Design review of the part built by this model. Coordinates are the model's own, in mm. A direction names the side the tool comes from. Coordinates: 2 decimals unless noted, no trailing zeros. Order: outer loops, then holes, each group sorted by start corner. A loop starts at its lowest first (then second) coordinate and runs counter-clockwise, first axis right, second up. Notation, with made-up numbers: (-33, 51) -> (5, 51) arc R23 ccw to (5, 69) -> close; hole circle Ø10 at (7.25, 44). An arc over 180 degrees is marked (long way). Write item = value, one per line.
Autodesk Inventor part; units mm, degrees
ref_plane "Work Plane1" through (0, 0, 48) normal (0, 0, 1) x (1, 0, 0)
ref_plane "YZ Plane" through (0, 0, 0) normal (1, 0, 0) x (0, 1, 0)
ref_plane "XZ Plane" through (0, 0, 0) normal (0, 1, 0) x (-1, 0, 0)
sketch "Sketch1" plane through (0, 0, 0) normal (0, 0, 1) x (1, 0, 0)
  line L0 (-19.05, 19.05) -> (19.05, 19.05)
  line L1 (19.05, 19.05) -> (19.05, -19.05)
  line L2 (19.05, -19.05) -> (-19.05, -19.05)
  line L3 (-19.05, -19.05) -> (-19.05, 19.05)
  point P0 (0, 0)
  point P1 (-19.05, 0)
  point P2 (0, 19.05)
  dimension "d0" = 38.1
extrude "Extrusion1" add sketch "Sketch1" along normal blind 56
sketch "Sketch2" plane through (-19.05, 19.05, 0) normal (0, 1, 0) x (1, 0, 0)
  circle A0 centre (19.05, -28) radius 12.7
  line L0 (0, 0) -> (38.1, 0)
  line L1 (0, -56) -> (38.1, -56)
  line L2 (17.05, 0) -> (21.05, 0)
  line L3 (21.05, 0) -> (21.05, -28)
  line L4 (21.05, -28) -> (17.05, -28)
  line L5 (17.05, -28) -> (17.05, 0)
  point P0 (19.05, 0)
  dimension "d3" = 28
  dimension "d4" = 25.4
  dimension "d5" = 4
extrude "Extrusion2" cut sketch "Sketch2" against normal through all
ref_plane "Work Plane1" through (0, 0, 48) normal (0, 0, 1) x (1, 0, 0)
sketch "Sketch3" plane through (0, 0, 48) normal (0, 0, 1) x (1, 0, 0)
  point P0 (0, 0)
hole "Hole1" at (0, 0, 48) direction (0, 0, 1) diameter 9 end through all
sketch "Sketch4" plane through (0, 0, 0) normal (0, 0, -1) x (-1, 0, 0)
  circle A0 centre (0, 0) radius 8
  dimension "d16" = 16
extrude "Extrusion3" cut sketch "Sketch4" against normal up to surface (48 mm away)
sketch "Sketch5" plane through (-19.05, -19.05, 0) normal (-1, 0, 0) x (0, 0, 1)
  line L0 (0, 0) -> (0, 38.1)
  circle A0 centre (5.7121, 19.05) radius 3.8228
  line L1 (4.9053, 27.6435) -> (6.5597, 27.6435)
  line L2 (6.5597, 27.6435) -> (6.5597, 10.4565)
  line L3 (6.5597, 10.4565) -> (4.9053, 10.4565)
  line L4 (4.9053, 10.4565) -> (4.9053, 27.6435)
  point P0 (0, 19.05)
  point P1 (6.5597, 19.05)
extrude "Extrusion4" add sketch "Sketch5" along normal blind 6
properties part number "22-134 Block"
(1) We need section C-C (x = 0). Write out the cut boundary in (y, z).
Report:
outline = (-19.05, 40.7) -> (-8, 40.7) -> (-8, 48) -> (-4.5, 48) -> (-4.5, 56) -> (-19.05, 56) -> close; (4.5, 48) -> (8, 48) -> (8, 40.7) -> (19.05, 40.7) -> (19.05, 56) -> (4.5, 56) -> close
(2) We need section A-A (y = 0). Write out the cut boundary in (x, z), and give its area (3 significant figures).
Report:
outline = (-25.05, 1.89) -> (-19.05, 1.89) -> (-19.05, 0) -> (-8, 0) -> (-8, 18.14) arc R12.7 cw to (-8, 37.86) -> (-8, 48) -> (-4.5, 48) -> (-4.5, 56) -> (-19.05, 56) -> (-19.05, 9.53) -> (-25.05, 9.53) -> close; (4.5, 48) -> (8, 48) -> (8, 37.86) arc R12.7 cw to (8, 18.14) -> (8, 0) -> (19.05, 0) -> (19.05, 56) -> (4.5, 56) -> close
area = 1,210 mm²
(3) For faces 4 (the flat face through (2, -13, 8)), 5 (the flat face through (-22, 8.594, 6)), 6 (the flat face through (-22, 6, 4.905)), list the 3-axis set-ups (+Z, -Z, +X, -X, +Y, -Y) from which the entire face can be reached by the end or side of a thin tool; tool diameter is ignored.
Report:
face_4 = -Z, +Y, -Y
face_5 = +Z, -Z, -X, +Y
face_6 = -Z, -X, +Y
(4) We need section D-D (z = 50.5). Write out the cut boundary in (x, y).
Report:
outline = (-19.05, -19.05) -> (19.05, -19.05) -> (19.05, 19.05) -> (-19.05, 19.05) -> close; hole circle Ø9 at (0, 0)
(5) Insertion check: pin 1 (10 mm diameter, centred on x = -7.5, z = 31, fed in from -Y); pin 2 (4 mm diameter, centred on y = -9, z = 43, fed in from -X); pin 3 (5 mm diameter, centred on x = 2, y = 1.5, fed in from -Z); pin 4 (1.5 mm diameter, centred on x = -22.5, y = 6, fed in from +Z). Each pin has a flat end and moves straight along its axis. Give the tip position at first contact, or say it passes through.
Report:
pin_1 = -19.05
pin_2 = -19.05
pin_3 = 48
pin_4 = 6.56
(6) We need section B-B (z = 28). Write out the cut boundary in (x, y), and give its area (3 significant figures).
Report:
outline = (-19.05, -19.05) -> (-12.7, -19.05) -> (-12.7, 19.05) -> (-19.05, 19.05) -> close; (12.7, -19.05) -> (19.05, -19.05) -> (19.05, 19.05) -> (12.7, 19.05) -> close
area = 484 mm²
(7) The part is to be moulded in two halves that separate along Y. For faces 1 (the cylindrical face through (-8, 0, 9)), 2 (the cylindrical face through (-22.008, 0.072, 9.534)), 3 (the flat face through (-22, -6, 6.56)), say which applies: released by +Y, released by -Y, zero draft, split by the parting line, or undercut.
Report:
face_1 = undercut
face_2 = split by the parting line
face_3 = zero draft
(8) For L1, parallel to Y at x = 0, z = 49.5; L2, parallel to X at y = 0, z = 45; L3, parallel to X at y = -8, z = 28, list the stretches that pass through material, from the lowest coordinate up.
Report:
L1 = -19.05 to -4.5, 4.5 to 19.05
L2 = -19.05 to -8, 8 to 19.05
L3 = -19.05 to -12.7, 12.7 to 19.05
